The listing builds one solid part. Answer for the finished solid, in the listing's coordinates (mm). Face numbers are marked on the shaded views. Coordinates: 2 decimals unless noted, no trailing zeros. Order: outer loops, then holes, each group sorted by start corner. A loop starts at its lowest first (then second) coordinate and runs counter-clockwise, first axis right, second up. Notation, with made-up numbers: (-1, -4.5) -> (23, -4.5) arc R17 ccw to (23, 19.5) -> close; hole circle Ø10 at (15, -32.75). An arc over 180 degrees is marked (long way). Return JSON: item names as keys, results as strings.
```python
from build123d import *

# Parameters (mm, degrees)
SKETCH1_W                                 = 253.492
SKETCH1_H                                 = 457.2
BASE_FLANGE1_DEPTH                        = 1.9939
EDGE_FLANGE1_STRIP_W                      = 13.66774
EDGE_FLANGE1_STRIP_H                      = 1.9939
EDGE_FLANGE1_STRIP_CUT_DEPTH              = 457.2
EDGE_FLANGE1_STRIP_2_W                    = 13.66774
EDGE_FLANGE1_STRIP_2_H                    = 1.9939
EDGE_FLANGE1_STRIP_CUT_2_DEPTH            = 457.2
EDGE_FLANGE1_DEPTH                        = 457.2
EDGE_FLANGE1_BEND_DEPTH                   = 457.2
HOLE_FOR_1_4_SELF_CLINCHING_NUTS_S_SS_C_D = 8.7376
CUT_EXTRUDE1_DEPTH                        = 525.657828078
SKETCH16_W                                = 253.492
SKETCH16_H                                = 25.4
CUT_EXTRUDE2_DEPTH                        = 525.657828078
FILLET1_R                                 = 2.54


# Sheet-metal steps are written as plain solids
with BuildPart() as part:
    # Sketch1 → Base-Flange1 (new body)
    with BuildSketch(Plane(origin=(0, 0, 0), x_dir=(1, 0, 0), z_dir=(0, 1, 0))):
        with Locations((126.746, 228.6)):
            Rectangle(SKETCH1_W, SKETCH1_H)
    extrude(amount=-BASE_FLANGE1_DEPTH)

    # Edge-Flange1 strip (across the edge) → Edge-Flange1 strip cut (cut)
    with BuildSketch(Plane.XY.offset(-457.2)):
        with Locations((-1.9939, -0.99695)):
            Rectangle(EDGE_FLANGE1_STRIP_W, EDGE_FLANGE1_STRIP_H)
    extrude(amount=EDGE_FLANGE1_STRIP_CUT_DEPTH, mode=Mode.SUBTRACT)

    # Edge-Flange1 strip 2 (across the edge) → Edge-Flange1 strip cut 2 (cut)
    with BuildSketch(Plane(origin=(253.492, 0, 0), x_dir=(-1, 0, 0), z_dir=(0, 0, -1))):
        with Locations((-1.9939, -0.99695)):
            Rectangle(EDGE_FLANGE1_STRIP_2_W, EDGE_FLANGE1_STRIP_2_H)
    extrude(amount=EDGE_FLANGE1_STRIP_CUT_2_DEPTH, mode=Mode.SUBTRACT)

    # Edge-Flange1 section (across the edge) → Edge-Flange1 (add)
    with BuildSketch(Plane.XY.offset(-457.2)):
        with BuildLine():
            Line((0, 2.84607), (0, 42.4561))
            Line((0, 42.4561), (1.9939, 42.4561))
            Line((1.9939, 42.4561), (1.9939, 2.84607))
            ThreePointArc((1.9939, 2.84607), (2.827494603, 0.833594603), (4.83997, 0))
            Line((4.83997, 0), (4.83997, -1.9939))
            ThreePointArc((4.83997, -1.9939), (1.417594392, -0.576305608), (0, 2.84607))
        make_face()
    extrude(amount=EDGE_FLANGE1_DEPTH)

    # Edge-Flange1 section 2 (across the edge) → Edge-Flange1 bend (add)
    with BuildSketch(Plane(origin=(253.492, 0, 0), x_dir=(-1, 0, 0), z_dir=(0, 0, -1))):
        with BuildLine():
            Line((0, 2.84607), (0, 42.4561))
            Line((0, 42.4561), (1.9939, 42.4561))
            Line((1.9939, 42.4561), (1.9939, 2.84607))
            ThreePointArc((1.9939, 2.84607), (2.827494603, 0.833594603), (4.83997, 0))
            Line((4.83997, 0), (4.83997, -1.9939))
            ThreePointArc((4.83997, -1.9939), (1.417594392, -0.576305608), (0, 2.84607))
        make_face()
    extrude(amount=EDGE_FLANGE1_BEND_DEPTH)

    # Hole for 1/4 Self-clinching Nuts (S,SS,CLS,CLSS)1 (through all)
    with Locations(Plane.ZY):
        with Locations((-406.4, 25.4), (-50.8, 25.4), (-381, 25.4), (-273.05, 25.4)):
            Hole(HOLE_FOR_1_4_SELF_CLINCHING_NUTS_S_SS_C_D / 2)

    # Sketch15 → Cut-Extrude1 (cut, through all)
    with BuildSketch(Plane.XZ.offset(1.9939)):
        with BuildLine():
            Line((215.646, -457.2), (37.846, -457.2))
            ThreePointArc((37.846, -457.2), (126.746, -419.1), (215.646, -457.2))
        make_face()
    extrude(amount=-CUT_EXTRUDE1_DEPTH, mode=Mode.SUBTRACT)

    # Sketch16 → Cut-Extrude2 (cut, through all)
    with BuildSketch(Plane.XZ.offset(1.9939)):
        with Locations((126.746, -444.5)):
            Rectangle(SKETCH16_W, SKETCH16_H)
    extrude(amount=-CUT_EXTRUDE2_DEPTH, mode=Mode.SUBTRACT)

    # Fillet1
    fillet1_edges = [part.edges().sort_by_distance(p)[0] for p in [
        (0.99695, 42.4561, -431.8),
        (252.49505, 42.4561, -431.8),
        (0.99695, 42.4561, 0),
        (252.49505, 42.4561, 0),
    ]]
    fillet(fillet1_edges, radius=FILLET1_R)


solid = part.part
```
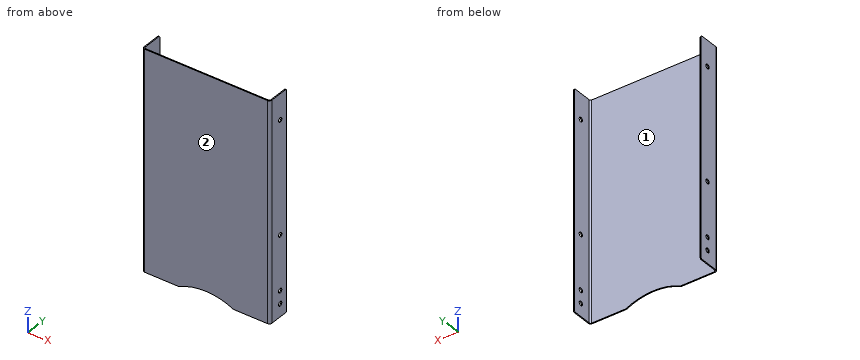
Item 1: The part is cut by section C-C on x = 63. Determine the outline of the cut face in (y, z), plus the area to 3 significant figures.
Answer list:
{"outline": "(-1.99, -431.8) -> (0, -431.8) -> (0, 0) -> (-1.99, 0) -> close", "area": "861 mm2"}
Item 2: The part is cut by section B-B on z = -50.8. Determine the outline of the cut face in (x, y).
Answer list:
{"outline": "(0, 2.85) arc R4.84 ccw to (4.84, -1.99) -> (248.65, -1.99) arc R4.84 ccw to (253.49, 2.85) -> (253.49, 21.03) -> (251.5, 21.03) -> (251.5, 2.85) arc R2.85 cw to (248.65, 0) -> (4.84, 0) arc R2.85 cw to (1.99, 2.85) -> (1.99, 21.03) -> (0, 21.03) -> close; (0, 29.77) -> (1.99, 29.77) -> (1.99, 42.46) -> (0, 42.46) -> close; (251.5, 29.77) -> (253.49, 29.77) -> (253.49, 42.46) -> (251.5, 42.46) -> close"}
Item 3: Flat-ended cylindrical pins translate along their axes: pin 1 (14 mm diameter, centred on y = 25.4, z = -381, fed in from -X); pin 2 (8 mm diameter, centred on x = 132, z = -147.5, fed in from +Y). Find the tip coordinate at first contact, or state that the pin passes through.
Answer list:
{"pin 1": "x = 0", "pin 2": "y = 0"}
Item 4: Find the intervals of material crossed by probe 1 along X at (y, z) = (36.5, -128); probe 2 along Y at (x, z) = (238.5, -263.5); probe 3 along Y at (x, z) = (252.45, -406.4), in increasing order.
Answer list:
{"probe 1": "0 to 1.99, 251.5 to 253.49", "probe 2": "-1.99 to 0", "probe 3": "-0.15 to 21.03, 29.77 to 42.46"}
Item 5: Determine the mould class of the marked faces 1 and 2 for opening direction X: pulls with the +X half, pulls with the -X half, needs draft (parallel to the pull), parting line crosses it, or undercut.
Answer list:
{"face 1": "undercut", "face 2": "needs draft"}
Item 6: The part is cut by section A-A on y = 9.5. Determine the outline of the cut face in (x, z), plus the area to 3 significant figures.
Answer list:
{"outline": "(0, -431.8) -> (1.99, -431.8) -> (1.99, 0) -> (0, 0) -> close; (251.5, -431.8) -> (253.49, -431.8) -> (253.49, 0) -> (251.5, 0) -> close", "area": "1,720 mm2"}
